```python
from build123d import *

# Parameters (mm, degrees)
F0_W     = 19.05
F0_H     = 3.429
F2_W     = 17.526
F2_H     = 2.413
F4_W     = 16.002
F4_H     = 2.413
F6_R     = 1.7399
F7_DEPTH = 6.985
F9_DEPTH = 2.54


with BuildPart() as f1:
    # F0 (on Front) → F1 (revolve)
    with BuildSketch(Plane.XZ):
        with Locations((9.525, 1.7145)):
            Rectangle(F0_W, F0_H)
    revolve(axis=Axis((0, 0, 1.7145), (0, 0, 1)))

    # F2 (on Front) → F3 (revolve)
    with BuildSketch(Plane.XZ):
        with Locations((8.763, 4.6355)):
            Rectangle(F2_W, F2_H)
    revolve(axis=Axis((0, 0, 4.6355), (0, 0, 1)))

    # F4 (on Front) → F5 (revolve)
    with BuildSketch(Plane.XZ):
        with Locations((8.001, 7.0485)):
            Rectangle(F4_W, F4_H)
    revolve(axis=Axis((0, 0, 7.0485), (0, 0, 1)))

    # F6 (on face) → F7 (cut)
    with BuildSketch(Plane.XY.offset(8.255)):
        with Locations((8.243714, 4.308599)):
            Circle(F6_R)
    extrude(amount=-F7_DEPTH, mode=Mode.SUBTRACT)

    # F8 (on face) → F9 (cut)
    with BuildSketch(Plane.XY.offset(8.255)):
        Polygon((10.986907, 4.302744), (9.620381, 6.681347), (6.877187, 6.687202), (5.50052, 4.314454), (6.867046, 1.935851), (9.61024, 1.929996), align=None)
    extrude(amount=-F9_DEPTH, mode=Mode.SUBTRACT)


solid = f1.part
```
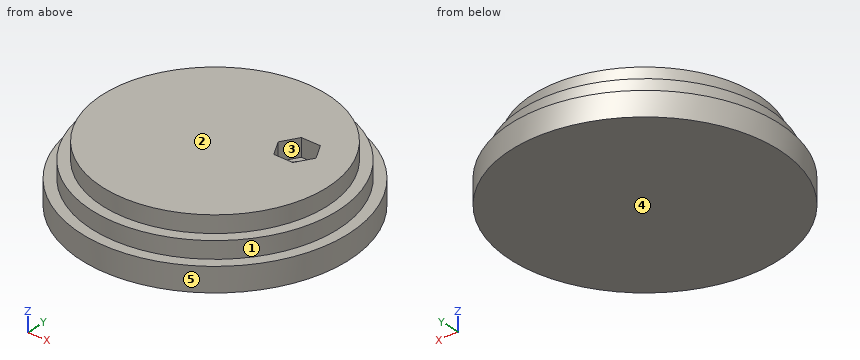
Could you check a few things on this model? Use its own coordinates, in mm. Face numbers are marked on the shaded views. A direction names the side the tool comes from. Coordinates: 2 decimals unless noted, no trailing zeros. Loops run counter-clockwise (first coordinate to the right, second up) from the corner with the lowest first, then second, coordinate; pieces in that order, holes last.
1) Which directions (+Z, -Z, +X, -X, +Y, -Y) give clear straight access to the entire face, cutting with the end or side of a thin tool? Please do the marked faces 1 and 2.
Reported:
face 1: +Z
face 2: +Z, +X, -X, +Y, -Y
2) Imagine slicing it at A-A (z = 7.5). List the corners of the cut face in (x, y) for me, and give its area (3 significant figures).
Reported:
outline: circle Ø32 at (0, 0); hole (5.5, 4.31) - (6.87, 1.94) - (9.61, 1.93) - (10.99, 4.3) - (9.62, 6.68) - (6.88, 6.69) - close
area: 785 mm2
3) Thinking about a two-plate mould opening in Y: for the marked faces 3, 4 and 5, which applies, released by +Y, released by -Y, zero draft, split by the parting line, or undercut?
Reported:
face 3: undercut
face 4: zero draft
face 5: split by the parting line
4) Imagine slicing it at B-B (x = 0). List the corners of the cut face in (y, z) for me (3 decimals).
Reported:
outline: (-19.05, 0) - (19.05, 0) - (19.05, 3.429) - (17.526, 3.429) - (17.526, 5.842) - (16.002, 5.842) - (16.002, 8.255) - (-16.002, 8.255) - (-16.002, 5.842) - (-17.526, 5.842) - (-17.526, 3.429) - (-19.05, 3.429) - close
5) Will these pins go through, and if not, where does the flat tip stop? pin 1 Ø2.5 at (x, y) = (7.5, 3.5) entering from +Z (3 decimals); pin 2 Ø4 at (x, z) = (-5.5, 7) entering from +Y; pin 3 Ø4 at (x, z) = (-0.5, 5) entering from +Y.
Reported:
pin 1: stops at z = 5.715
pin 2: stops at y = 17.09
pin 3: stops at y = 19.05
6) Please list where these lines run through material, in increasing order: line 1 along Z through (x, y) = (14, 11); line 2 along Z through (x, y) = (17, -2); line 3 along Y through (x, z) = (6, 6.75).
Reported:
line 1: z = 0 to 3.43
line 2: z = 0 to 5.84
line 3: y = -14.83 to 3.45, 5.18 to 14.83
7) Imagine slicing it at C-C (y = -1). List the corners of the cut face in (x, z) for me (3 decimals), and give its area (3 significant figures).
Reported:
outline: (-19.024, 0) - (19.024, 0) - (19.024, 3.429) - (17.497, 3.429) - (17.497, 5.842) - (15.971, 5.842) - (15.971, 8.255) - (-15.971, 8.255) - (-15.971, 5.842) - (-17.497, 5.842) - (-17.497, 3.429) - (-19.024, 3.429) - close
area: 292 mm2
